```python
from build123d import *

# Parameters (mm, degrees)
BOSS_EXTRUDE1_DEPTH   = 10
F_8_0MM_DOWEL_HOLE1_D = 8


with BuildPart() as part:
    # Sketch1 → Boss-Extrude1 (new body)
    with BuildSketch(Plane.XY):
        Polygon((-23.981742881, 0), (23.981742881, 0), (23.981742881, 17.869578459), (10.906262583, 38.719668664), (7.5, 38.719668664), (7.5, 15.649448466), (-7.5, 15.649448466), (-7.5, 38.719668664), (-10.906262583, 38.719668664), (-23.981742881, 17.869578459), align=None)
    extrude(amount=BOSS_EXTRUDE1_DEPTH)

    # Ø8.0mm Dowel Hole1 (through all)
    with Locations(Plane(origin=(0, 0, 0), x_dir=(-1, 0, 0), z_dir=(0, -1, 0))):
        with Locations((10, -5.102347766), (-10, -5.102347766)):
            Hole(F_8_0MM_DOWEL_HOLE1_D / 2)


solid = part.part
```
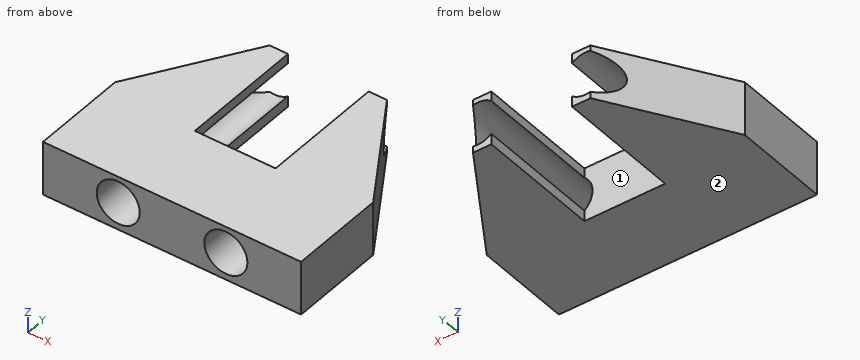
Verification items for the finished model (mm, model axes). Face numbers are marked on the shaded views. A direction names the side the tool comes from. Give positions to 0.01 mm unless a question says otherwise; leave off trailing zeros. Loops run counter-clockwise (first coordinate to the right, second up) from the corner with the lowest first, then second, coordinate; pieces in that order, holes last. Notation, with made-up numbers: M 23,27.25 L 50,27.25 A14 cw 50,51.25 Z; hole C 67.25,14 d11. An arc over 180 degrees is marked long. Return JSON: item names as keys, results as strings.
1) Tool access check on the marked faces 1 and 2. Record the directions out of +Z, -Z, +X, -X, +Y, -Y that give a thin tool (end or side, any length) a straight path to the whole face; none if there is none.
Findings:
{"face 1": "+Z, -Z, +Y", "face 2": "-Z, +X, -X, +Y, -Y"}
2) Material ranges on L1, parallel to Z at x = -10, y = 26.5; L2, parallel to X at y = 2, z = 6.5; L3, parallel to X at y = 4.5, z = 7.75, recorded low to high. Write a range as [from, to].
Findings:
{"L1": "z = [0, 1.1], [9.1, 10]", "L2": "x = [-23.98, -13.75], [-6.25, 6.25], [13.75, 23.98]", "L3": "x = [-23.98, -13], [-7, 7], [13, 23.98]"}
3) Section check D-D, the plane y = 9. Enter the section's corners in (x, z), and give its area (3 significant figures).
Findings:
{"outline": "M -23.98,0 L 23.98,0 L 23.98,10 L -23.98,10 Z; hole C -10,5.1 d8; hole C 10,5.1 d8", "area": "379 mm2"}
4) Gauge pin test, flat ends, axial feed: P1, Ø1, axis at y = 26, z = 0.5, coming from the -X side; P2, Ø0.9, axis at y = 26, z = 9.5, coming from the +X side; P3, Ø4, axis at x = -6, z = 6.5, coming from the +Y side. Record the tip position at first contact, or that the pin passes through.
Findings:
{"P1": "stops at x = -19.2", "P2": "stops at x = 19.17", "P3": "stops at y = 15.65"}
5) Section check A-A, the plane x = -10. Enter the section's corners in (y, z).
Findings:
{"outline": "M 0,0 L 38.72,0 L 38.72,1.1 L 0,1.1 Z; M 0,9.1 L 38.72,9.1 L 38.72,10 L 0,10 Z"}
6) Section check B-B, the plane z = 5.75. Enter the section's corners in (x, y).
Findings:
{"outline": "M -23.98,0 L -13.95,0 L -13.95,33.87 L -23.98,17.87 Z; M -6.05,0 L 6.05,0 L 6.05,15.65 L -6.05,15.65 Z; M 13.95,0 L 23.98,0 L 23.98,17.87 L 13.95,33.87 Z"}
7) Section check C-C, the plane y = 29.5. Enter the section's corners in (x, z), and give its area (3 significant figures).
Findings:
{"outline": "M -16.69,0 L -7.5,0 L -7.5,1.98 A4 cw long -7.5,8.22 L -7.5,10 L -16.69,10 Z; M 7.5,0 L 16.69,0 L 16.69,10 L 7.5,10 L 7.5,8.22 A4 cw long 7.5,1.98 Z", "area": "96.3 mm2"}
